Verification items for the finished model (mm, model axes). A direction names the side the tool comes from. Round coordinates to 2 decimals unless told otherwise and drop trailing zeros. Loops run counter-clockwise (first coordinate to the right, second up) from the corner with the lowest first, then second, coordinate; pieces in that order, holes last.
from build123d import *

# Parameters (mm, degrees)
F0_W     = 6.45
F0_H     = 6.45
F2_DEPTH = 12
F1_R     = 2.8
F3_DEPTH = 12
F4_W     = 0.8
F4_H     = 5.918589
F5_DEPTH = 12


with BuildPart() as f2:
    # F0 (on Front) → F2 (new body)
    with BuildSketch(Plane.XZ):
        Rectangle(F0_W, F0_H)
    extrude(amount=F2_DEPTH)

    # F1 (on Front) → F3 (cut)
    with BuildSketch(Plane.XZ):
        Circle(F1_R)
    extrude(amount=F3_DEPTH, mode=Mode.SUBTRACT)

    # F4 (on Front) → F5 (join)
    with BuildSketch(Plane.XZ):
        with Locations((-2.508641, 0.172032)):
            Rectangle(F4_W, F4_H)
    extrude(amount=F5_DEPTH)


solid = f2.part
1. Tool access check on faces 4 (the face through (3.225, -6, 0)), 5 (the face through (-2.109, -6, 0)). Record the directions out of +Z, -Z, +X, -X, +Y, -Y that give a thin tool (end or side, any length) a straight path to the whole face; none if there is none.
2. Release check for a two-part mould opening along X. For faces 1 (the face through (2.8, -5.9, -0.1)), 2 (the face through (-3, 0, 0)), 3 (the face through (-3.225, -6, 0)) record: released by +X, released by -X, zero draft, split by the parting line, or undercut.
3. Section check B-B (z = 0). Enter the section's corners in (x, y) (3 decimals).
4. Scan lines: L1, parallel to X at y = -2.5, z = 0 (3 decimals); L2, parallel to Z at x = 0, y = -9 (3 decimals); L3, parallel to Z at x = -2, y = -2 (3 decimals). Record each from-to range of solid material in increasing order.
5. Section check A-A (x = 0). Enter the section's corners in (y, z) (3 decimals), then the cut area to 3 significant figures.
6. Section check C-C (y = -2). Enter the section's corners in (x, z) (3 decimals).
Taken from the geometry:
1. face 4: +Z, -Z, +X, +Y, -Y
1. face 5: +Y, -Y
2. face 1: undercut
2. face 2: zero draft
2. face 3: released by -X
3. outline: (-3.225, -12) - (-2.109, -12) - (-2.109, 0) - (-3.225, 0) - close; (2.8, -12) - (3.225, -12) - (3.225, 0) - (2.8, 0) - close
4. L1: x = -3.225 to -2.109, 2.8 to 3.225
4. L2: z = -3.225 to -2.8, 2.8 to 3.225
4. L3: z = -3.225 to -1.96, 1.96 to 3.225
5. outline: (-12, -3.225) - (0, -3.225) - (0, -2.8) - (-12, -2.8) - close; (-12, 2.8) - (0, 2.8) - (0, 3.225) - (-12, 3.225) - close
5. area: 10.2 mm2
6. outline: (-3.225, -3.225) - (3.225, -3.225) - (3.225, 3.225) - (-3.225, 3.225) - close; hole (-2.109, -1.842) arc R2.8 ccw (long way) to (-2.109, 1.842) - close
